```python
from build123d import *

# Parameters (mm, degrees)
F0_R            = 44.45
F0_R_2          = 14.1605
F1_DEPTH        = 3.175
F2_R            = 2.3622
F3_DEPTH        = 3.176
F3_COPIES_COUNT = 6


# Not quite as in the source:
# - a pattern or mirror of a feature is missing from the dataset's text; its kind, count and spacing are read off the source's solid


with BuildPart() as f1:
    # F0 (on Top) → F1 (new body)
    with BuildSketch(Plane.XY):
        Circle(F0_R)
        Circle(F0_R_2, mode=Mode.SUBTRACT)
    extrude(amount=F1_DEPTH)

    # F2 (on face) → F3 (cut, through all)
    with BuildSketch(Plane.XY.offset(3.175)):
        with Locations((0, 23.8125)):
            Circle(F2_R)
    f3 = extrude(amount=-F3_DEPTH, mode=Mode.SUBTRACT)

    # F3_copies: F3 ×6 about axis
    f3_copies_axis = Axis((0, 0, 0), (0, 0, 1))
    for i in range(1, F3_COPIES_COUNT):
        add(f3.rotate(f3_copies_axis, i * 360 / F3_COPIES_COUNT), mode=Mode.SUBTRACT)


solid = f1.part
```
The model under review builds one solid part; all positions refer to its coordinate system, in mm. Coordinates: 2 decimals unless noted, no trailing zeros. Order: outer loops, then holes, each group sorted by start corner. A loop starts at its lowest first (then second) coordinate and runs counter-clockwise, first axis right, second up. Notation, with made-up numbers: M -19.75,-3 L 25.25,-3 A33 ccw 25.25,29 Z; hole C 50,0 d4. An arc over 180 degrees is marked long. One line per question, with ' | ' between items.
(1) Add section B-B, the plane x = 0. State how many separate pieces and enclosed holes the cut face has, then the cut area to 3 significant figures.
Geometry results:
separate pieces: 4 | enclosed holes: 0 | area: 162 mm²
(2) For probe 1 along Y at (x, z) = (0, 2.55); probe 2 along X at (y, z) = (-13, 2.25); probe 3 along X at (y, z) = (12, 2.6), list the stretches that pass through material, from the lowest coordinate up. Write a range as from..to.
Geometry results:
probe 1: y = -44.45..-26.17, -21.45..-14.16, 14.16..21.45, 26.17..44.45 | probe 2: x = -42.51..-22.72, -18.53..-5.61, 5.61..18.53, 22.72..42.51 | probe 3: x = -42.8..-22.98, -18.26..-7.52, 7.52..18.26, 22.98..42.8
(3) Add section C-C, the plane z = 2.2. Write out the cut boundary in (x, y).
Geometry results:
outline: C 0,0 d88.9; hole C -20.62,-11.91 d4.72; hole C -20.62,11.91 d4.72; hole C 0,0 d28.32; hole C 0,-23.81 d4.72; hole C 0,23.81 d4.72; hole C 20.62,-11.91 d4.72; hole C 20.62,11.91 d4.72
(4) The part is to be moulded in two halves that separate along X. For faces 1 (the face through (22.875, -11.197, 1.61)), 2 (the face through (-11, 11, 0)), 3 (the face through (42.397, 13.352, 1.565)), say which applies: +X half, -X half, draft (parallel to the pull), parting line (faces both ways), or undercut.
Geometry results:
face 1: undercut | face 2: draft | face 3: parting line
(5) Add section D-D, the plane x = -10.5. Write out the cut boundary in (y, z) (3 decimals), then the cut area to 3 significant figures.
Geometry results:
outline: M -43.192,0 L -9.501,0 L -9.501,3.175 L -43.192,3.175 Z; M 9.501,0 L 43.192,0 L 43.192,3.175 L 9.501,3.175 Z | area: 214 mm²
(6) Insertion check: pin 1 (1.5 mm diameter, centred on x = 4.5, z = 1.5, fed in from +Y); pin 2 (3 mm diameter, centred on x = 0, y = 23.81, fed in from +Z); pin 3 (1 mm diameter, centred on x = 14.5, z = 2.5, fed in from +Y); pin 4 (1.5 mm diameter, centred on x = -27, z = 2.5, fed in from +Y). Each pin has a flat end and moves straight along its axis. Give the tip position at first contact, or say it passes through.
Geometry results:
pin 1: stops at y = 44.29 | pin 2: passes through | pin 3: stops at y = 42.19 | pin 4: stops at y = 35.87
